Build history of the part. All positions in model axes, mm. A direction names the side the tool comes from. Give positions to 0.01 mm unless a question says otherwise; leave off trailing zeros. Loops run counter-clockwise (first coordinate to the right, second up) from the corner with the lowest first, then second, coordinate; pieces in that order, holes last. Notation, with made-up numbers: (-7, 40.25) -> (-3, 40.25) arc R14 ccw to (-3, 58.25) -> close; hole circle Ø7 at (30.25, 11). An arc over 180 degrees is marked (long way). One line per question, with ' | ' between items. Start each with the question number.
(1) Slice it at C-C, the plane x = 21. Write the cut outline in (y, z), then the cut area to 3 significant figures.
(2) Slice it at A-A, the plane x = 35. Write the cut outline in (y, z).
(3) 3-axis set-ups, long thin cutter, end or side, ignore diameter. For faces 4 (the face through (65, 13, -69)), 5 (the face through (4, 13, -69)), 6 (the face through (35, 8, -22)), 7 (the face through (35, 0, -28)), 8 (the face through (35, 10, -77)): which of +Z, -Z, +X, -X, +Y, -Y reach the whole face in a straight line?
(4) Slice it at D-D, the plane z = -9. Write the cut outline in (x, y), then the cut area to 3 significant figures.
(5) Drill centre lines: L1, parallel to Y at x = 35, z = -66; L2, parallel to Y at x = 35, z = -72; L3, parallel to Z at x = 26, y = 22.5. Where is each one in solid material? Low to high. Write a range as from..to.
(6) Flat gauge pins, fed straight in: pin 1 Ø0.6 at (x, y) = (34.5, 9.5) entering from +Z; pin 2 Ø8 at (x, z) = (21.5, -1) entering from +Y; pin 3 Ø3 at (y, z) = (6.5, -51.5) entering from +X. Where does each tip first touch, or does it go through?
(7) Slice it at B-B, the plane y = 20. Write the cut outline in (x, z).
(8) Mould opens along X. For faces 1 (the face through (70, 21, -69)), 2 (the face through (32, 23, -70.014)), 3 (the face through (35, 26, -74.014)) say: pulls with the +X half, pulls with the -X half, needs draft (parallel to the pull), parting line crosses it, or undercut.
```python
from build123d import *

# Parameters (mm, degrees)
EXTRUDE_1_DEPTH     = 70
CUT_EXTRUDE_1_DEPTH = 163
SKETCH_3_W          = 5
SKETCH_3_H          = 28.984249348
CUT_EXTRUDE_2_DEPTH = 74.198677084
SKETCH_4_W          = 20.259313124
SKETCH_4_H          = 10.192966915
CUT_EXTRUDE_3_DEPTH = 77.198677084
SKETCH_5_W          = 22.578654877
SKETCH_5_H          = 21
CUT_EXTRUDE_4_DEPTH = 77
SKETCH_7_R          = 6
CUT_EXTRUDE_5_DEPTH = 37
SKETCH_8_R          = 8
CUT_EXTRUDE_6_DEPTH = 4


with BuildPart() as part:
    # Эскиз1 → Бобышка-Вытянуть1 (new body)
    with BuildSketch(Plane(origin=(0, 0, 0), x_dir=(0, 0, -1), z_dir=(1, 0, 0))):
        with BuildLine():
            Line((-20.986257223, 0), (79.013742777, 0))
            Line((79.013742777, 0), (79.013742777, 32))
            ThreePointArc((79.013742777, 32), (77.549276683, 35.535533906), (74.013742777, 37))
            Line((74.013742777, 37), (71.922596638, 37))
            ThreePointArc((71.922596638, 37), (69.613853571, 36.435054166), (67.826836416, 34.867882182))
            Line((67.826836416, 34.867882182), (49.013742777, 8))
            Line((49.013742777, 8), (-20.986257223, 8))
            Line((-20.986257223, 8), (-20.986257223, 0))
        make_face()
    extrude(amount=EXTRUDE_1_DEPTH)

    # Эскиз2 → Вырез-Вытянуть1 (cut)
    with BuildSketch(Plane(origin=(0, 0, -79.013742777), x_dir=(-1, 0, 0), z_dir=(0, 0, -1))):
        Polygon((-61, 13), (-70, 13), (-70, 0), (-60.293754471, 11.56745298), align=None)
        Polygon((-9, 13), (-9.706245529, 11.56745298), (0, 0), (0, 13), align=None)
    extrude(amount=-CUT_EXTRUDE_1_DEPTH, mode=Mode.SUBTRACT)

    # Эскиз3 → Вырез-Вытянуть2 (cut)
    with BuildSketch(Plane.ZY):
        with Locations((-76.513742777, 24.492124674)):
            Rectangle(SKETCH_3_W, SKETCH_3_H)
    extrude(amount=-CUT_EXTRUDE_2_DEPTH, mode=Mode.SUBTRACT)

    # Эскиз4 → Вырез-Вытянуть3 (cut)
    with BuildSketch(Plane.ZY):
        with Locations((-65.118798198, 34.096483457)):
            Rectangle(SKETCH_4_W, SKETCH_4_H)
    extrude(amount=-CUT_EXTRUDE_3_DEPTH, mode=Mode.SUBTRACT)

    # Эскиз5 → Вырез-Вытянуть4 (cut)
    with BuildSketch(Plane(origin=(70, 0, 0), x_dir=(0, 0, -1), z_dir=(1, 0, 0))):
        with Locations((52.428773641, 18.5)):
            Rectangle(SKETCH_5_W, SKETCH_5_H)
    extrude(amount=-CUT_EXTRUDE_4_DEPTH, mode=Mode.SUBTRACT)

    # Эскиз7 → Вырез-Вытянуть5 (cut)
    with BuildSketch(Plane(origin=(0, 0, -74.013742777), x_dir=(-1, 0, 0), z_dir=(0, 0, -1))):
        with Locations((-35, 17.436066506)):
            Circle(SKETCH_7_R)
    extrude(amount=-CUT_EXTRUDE_5_DEPTH, mode=Mode.SUBTRACT)

    # Эскиз8 → Вырез-Вытянуть6 (cut)
    with BuildSketch(Plane(origin=(0, 0, -74.013742777), x_dir=(-1, 0, 0), z_dir=(0, 0, -1))):
        with Locations((-35, 17.436066506)):
            Circle(SKETCH_8_R)
    extrude(amount=-CUT_EXTRUDE_6_DEPTH, mode=Mode.SUBTRACT)


solid = part.part
```
Final values:
1) outline: (0, -79.01) -> (10, -79.01) -> (10, -74.01) -> (29, -74.01) -> (29, -63.72) -> (8, -63.72) -> (8, 20.99) -> (0, 20.99) -> close | area: 1,030 mm2
2) outline: (0, -79.01) -> (10, -79.01) -> (10, -74.01) -> (9.44, -74.01) -> (9.44, -70.01) -> (11.44, -70.01) -> (11.44, -63.72) -> (8, -63.72) -> (8, 20.99) -> (0, 20.99) -> close; (23.44, -70.01) -> (25.44, -70.01) -> (25.44, -74.01) -> (29, -74.01) -> (29, -63.72) -> (23.44, -63.72) -> close
3) face 4: +Z, -Z, +X | face 5: +Z, -Z, -X | face 6: +Z, +X, -X, +Y | face 7: +Z, -Z, +X, -X, -Y | face 8: -Z, +X, -X, +Y
4) outline: (0, 0) -> (70, 0) -> (63.29, 8) -> (6.71, 8) -> close | area: 506 mm2
5) L1: 0..11.44, 23.44..29 | L2: 0..9.44, 25.44..29 | L3: -74.01..-63.72
6) pin 1: z = -63.72 | pin 2: y = 8 | pin 3: x = 65.8
7) outline: (0, -74.01) -> (27.42, -74.01) -> (27.42, -70.01) -> (29.58, -70.01) -> (29.58, -63.72) -> (0, -63.72) -> close; (40.42, -70.01) -> (42.58, -70.01) -> (42.58, -74.01) -> (70, -74.01) -> (70, -63.72) -> (40.42, -63.72) -> close
8) face 1: pulls with the +X half | face 2: undercut | face 3: needs draft
